from build123d import *

# Parameters (mm, degrees)
BOSS_EXTRUDE1_DEPTH = 2
SKETCH4_R           = 1.5
CUT_EXTRUDE1_DEPTH  = 3


with BuildPart() as part:
    # Sketch1 → Boss-Extrude1 (new body)
    with BuildSketch(Plane(origin=(0, 0, 0), x_dir=(1, 0, 0), z_dir=(0, 1, 0))):
        with BuildLine():
            Line((-687.300884956, 62.644247788), (-814.660884956, 62.644247788))
            ThreePointArc((-814.660884956, 62.644247788), (-818.196418862, 61.179781694), (-819.660884956, 57.644247788))
            Line((-819.660884956, 57.644247788), (-819.660884956, 7.644247788))
            ThreePointArc((-819.660884956, 7.644247788), (-818.196418862, 4.108713882), (-814.660884956, 2.644247788))
            Line((-814.660884956, 2.644247788), (-687.300884956, 2.644247788))
            ThreePointArc((-687.300884956, 2.644247788), (-683.76535105, 4.108713882), (-682.300884956, 7.644247788))
            Line((-682.300884956, 7.644247788), (-682.300884956, 57.644247788))
            ThreePointArc((-682.300884956, 57.644247788), (-683.76535105, 61.179781694), (-687.300884956, 62.644247788))
        make_face()
    extrude(amount=BOSS_EXTRUDE1_DEPTH)

    # Sketch4 → Cut-Extrude1 (cut, through all)
    with BuildSketch(Plane.XZ):
        with Locations((-811.660884956, -10.644247788)):
            Circle(SKETCH4_R)
        with Locations((-811.660884956, -45.644247788)):
            Circle(SKETCH4_R)
        with Locations((-690.300884956, -10.644247788)):
            Circle(SKETCH4_R)
        with Locations((-690.300884956, -45.644247788)):
            Circle(SKETCH4_R)
    extrude(amount=-CUT_EXTRUDE1_DEPTH, mode=Mode.SUBTRACT)


solid = part.part
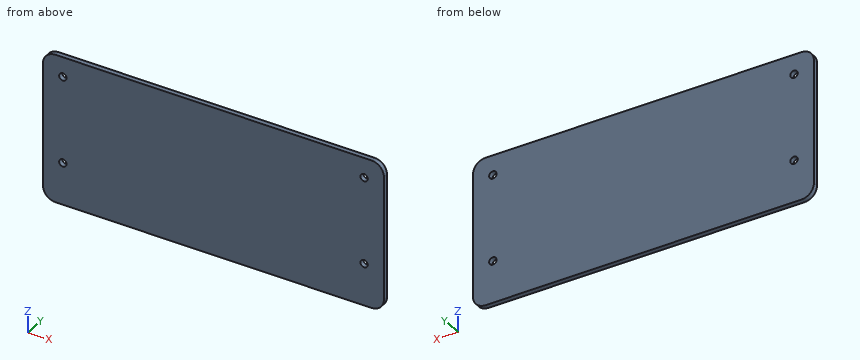
Verification items for the finished model (mm, model axes). Coordinates: 2 decimals unless noted, no trailing zeros. Loops run counter-clockwise (first coordinate to the right, second up) from the corner with the lowest first, then second, coordinate; pieces in that order, holes last. Notation, with made-up numbers: (-12, 40) -> (-2, 40) arc R16 ccw to (-2, 69) -> close; hole circle Ø11 at (70, 16.5). An arc over 180 degrees is marked (long way). Answer as a JSON object with one key per item and string values. Group by question number.
Item 1: Scan lines: probe 1 along X at (y, z) = (1.05, -45.5); probe 2 along X at (y, z) = (1.25, -45); probe 3 along X at (y, z) = (0.6, -7). Record each from-to range of solid material in increasing order.
Item 2: Depth check by flat-ended pin: pin 1 (2.5 mm diameter, centred on x = -811.66, z = -10.64, fed in from +Y); pin 2 (3.5 mm diameter, centred on x = -690.3, z = -10.64, fed in from -Y). Enter the tip coordinate at first touch or a pass-through.
Item 3: Sectioned sample at A-A on x = -690.5. Record the boundary of the cut face in (y, z), plus the area to 3 significant figures.
Evaluation:
{
 "1": {"probe 1": "x = -819.66 to -813.15, -810.17 to -691.79, -688.81 to -682.3", "probe 2": "x = -819.66 to -813.02, -810.31 to -691.66, -688.95 to -682.3", "probe 3": "x = -819.62 to -682.34"},
 "2": {"pin 1": "passes through", "pin 2": "stops at y = 0"},
 "3": {"outline": "(0, -62.64) -> (2, -62.64) -> (2, -47.13) -> (0, -47.13) -> close; (0, -44.16) -> (2, -44.16) -> (2, -12.13) -> (0, -12.13) -> close; (0, -9.16) -> (2, -9.16) -> (2, -2.64) -> (0, -2.64) -> close", "area": "108 mm²"}
}
